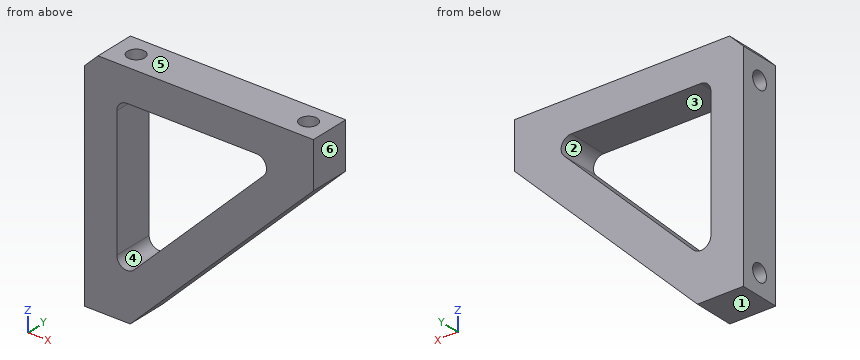
```python
from build123d import *

# Parameters (mm, degrees)
BOSS_EXTRUDE1_DEPTH           = 6.35
FILLET1_R                     = 1.588
TAP_DRILL_FOR_6_32_TAP2_D     = 2.7051
TAP_DRILL_FOR_6_32_TAP2_DEPTH = 6.35
TAP_DRILL_FOR_6_32_TAP2_TIP   = 0.81269403
TAP_DRILL_FOR_6_32_TAP1_D     = 2.7051
TAP_DRILL_FOR_6_32_TAP1_DEPTH = 6.35
TAP_DRILL_FOR_6_32_TAP1_TIP   = 0.81269403
CHAMFER1_SIZE                 = 2.155


with BuildPart() as part:
    # Sketch1 → Boss-Extrude1 (new body)
    with BuildSketch(Plane(origin=(0, 0, 0), x_dir=(1, 0, 0), z_dir=(0, 1, 0))):
        Polygon((0, 0), (0, 35.814), (7.183953537, 35.814), (35.814, 7.183953537), (35.814, 0), align=None)
        Polygon((5.08, 30.73374864), (5.08, 5.08), (30.73374864, 5.08), align=None, mode=Mode.SUBTRACT)
    extrude(amount=BOSS_EXTRUDE1_DEPTH)

    # Fillet1
    fillet1_edges = [part.edges().sort_by_distance(p)[0] for p in [
        (30.73374864, 3.175, -5.08),
        (5.08, 3.175, -30.73374864),
        (5.08, 3.175, -5.08),
    ]]
    fillet(fillet1_edges, radius=FILLET1_R)

    # Tap Drill for #6-32 Tap2
    with Locations(Plane.ZY):
        with Locations((-5.588, 3.175), (-32.5374, 3.175)):
            Hole(TAP_DRILL_FOR_6_32_TAP2_D / 2, depth=TAP_DRILL_FOR_6_32_TAP2_DEPTH)
            with Locations((0, 0, -(TAP_DRILL_FOR_6_32_TAP2_DEPTH + TAP_DRILL_FOR_6_32_TAP2_TIP / 2))):  # 118° drill point
                Cone(0, TAP_DRILL_FOR_6_32_TAP2_D / 2, TAP_DRILL_FOR_6_32_TAP2_TIP, mode=Mode.SUBTRACT)

    # Tap Drill for #6-32 Tap1
    with Locations(Plane.XY):
        with Locations((32.5374, 3.175), (5.588, 3.175)):
            Hole(TAP_DRILL_FOR_6_32_TAP1_D / 2, depth=TAP_DRILL_FOR_6_32_TAP1_DEPTH)
            with Locations((0, 0, -(TAP_DRILL_FOR_6_32_TAP1_DEPTH + TAP_DRILL_FOR_6_32_TAP1_TIP / 2))):  # 118° drill point
                Cone(0, TAP_DRILL_FOR_6_32_TAP1_D / 2, TAP_DRILL_FOR_6_32_TAP1_TIP, mode=Mode.SUBTRACT)

    # Chamfer1
    chamfer1_edges = [part.edges().sort_by_distance(p)[0] for p in [
        (0, 3.175, 0),
    ]]
    chamfer(chamfer1_edges, length=CHAMFER1_SIZE)


solid = part.part
```
The listing builds one solid part. Answer for the finished solid, in the listing's coordinates (mm). Face numbers are marked on the shaded views. A direction names the side the tool comes from. Give positions to 0.01 mm unless a question says otherwise; leave off trailing zeros. Write each loop counter-clockwise with the first axis right and the second up, starting at its lowest first coordinate (ties: lowest second). Pieces come first, ordered by that corner, then holes. Notation, with made-up numbers: (52, -29) - (73, -29) arc R30 ccw to (73, 7) - close; hole circle Ø10 at (-27, 87.25). An arc over 180 degrees is marked (long way). Use one line per item in the form item = value. Start each with the question number.
1) The mould has two halves that part along Z. Classify the marked faces 3, 4, 5 and 6: pulls with the +Z half, pulls with the -Z half, needs draft (parallel to the pull), parting line crosses it, or undercut.
2) Find section D-D on z = -3. Determine the outline of the cut face in (x, y) (3 decimals), plus the area to 3 significant figures.
3) Flat-ended cylindrical pins translate along their axes: pin 1 Ø1.6 at (y, z) = (3.18, -32.54) entering from +X; pin 2 Ø2 at (x, y) = (32.54, 3.18) entering from +Z; pin 3 Ø1.6 at (x, y) = (5.588, 3.175) entering from +Z. Find the tip coordinate at first contact, or state that the pin passes through.
4) Find section C-C on x = 11. Determine the outline of the cut face in (y, z).
5) A tool of negligible diameter and unlimited length cuts with its end or side. For the marked faces 1 and 2, from which of +Z, -Z, +X, -X, +Y, -Y can it reach the whole face along a straight path? Write none if from no direction.
6) Find section A-A on y = 5.5. Determine the outline of the cut face in (x, z) (3 decimals).
7) Find section B-B on z = -12. Determine the outline of the cut face in (x, y).
8) Consider line 1 along Z through (x, y) = (27.5, 4.75); line 2 along Z through (x, y) = (22, 2.5); line 3 along X through (y, z) = (5.25, -20). Determine where each line is inside the solid, lowest interval first. Write a range as from..to.
Geometry results:
q1.face_3 = undercut
q1.face_4 = undercut
q1.face_5 = pulls with the +Z half
q1.face_6 = needs draft
q2.outline = (0, 0) - (35.814, 0) - (35.814, 6.35) - (0, 6.35) - close; hole circle Ø2.705 at (5.588, 3.175); hole circle Ø2.705 at (32.537, 3.175)
q2.area = 216 mm2
q3.pin_1 = 11.26
q3.pin_2 = -6.56
q3.pin_3 = -6.79
q4.outline = (0, -32) - (6.35, -32) - (6.35, -24.81) - (0, -24.81) - close; (0, -5.08) - (6.35, -5.08) - (6.35, 0) - (0, 0) - close
q5.face_1 = -Z, +X, -X, +Y, -Y
q5.face_2 = +Y, -Y
q6.outline = (0, -35.814) - (7.184, -35.814) - (35.814, -7.184) - (35.814, 0) - (2.155, 0) - (0, -2.155) - close; hole (5.08, -26.9) arc R1.588 ccw to (7.791, -28.023) - (28.023, -7.791) arc R1.588 ccw to (26.9, -5.08) - (6.668, -5.08) arc R1.588 ccw to (5.08, -6.668) - close
q7.outline = (0, 0) - (5.08, 0) - (5.08, 6.35) - (0, 6.35) - close; (23.81, 0) - (31, 0) - (31, 6.35) - (23.81, 6.35) - close
q8.line_1 = -15.5..-8.31, -5.2..0
q8.line_2 = -21..-13.81, -5.08..0
q8.line_3 = 0..5.08, 15.81..23
